```python
from build123d import *

# Parameters (mm, degrees)
F1_DEPTH = 75
F2_W     = 28
F2_H     = 5.4
F2_W_2   = 28.1193151165
F2_H_2   = 5.3996254659
F2_W_3   = 28.3288413435
F2_H_3   = 5.3951430639
F2_W_4   = 28.8207556829
F2_W_5   = 28.5256083831
F2_H_4   = 5.4125102987
F2_W_6   = 29.607820116
F2_W_7   = 29.9029674158
F3_DEPTH = 2.8
F5_DEPTH = 5
F6_R     = 1.6
F7_DEPTH = 3.101
F8_SIZE  = 2
F9_R     = 0.5


with BuildPart() as f1:
    # F0 (on Front) → F1 (new body, symmetric)
    with BuildSketch(Plane.XZ):
        Polygon((-7.5, -4.8), (7.5, -4.8), (7.5, -3), (10.5, 0.3), (7.5, 3.3), (-7.5, 3.3), (-10.5, 0.3), (-7.5, -3), align=None)
    extrude(amount=F1_DEPTH, both=True)

    # F2 (on face) → F3 (cut)
    with BuildSketch(Plane.XY.offset(3.3)):
        Rectangle(F2_W, F2_H)
        with Locations((0.0596575582, 9.8198127329)):
            Rectangle(F2_W_2, F2_H_2)
        with Locations((0.1644206718, 19.6375715319)):
            Rectangle(F2_W_3, F2_H_3)
        with Locations((0.4103778414, 29.46)):
            Rectangle(F2_W_4, F2_H)
        with Locations((0.2628041916, -9.8137448507)):
            Rectangle(F2_W_5, F2_H_4)
        with Locations((0.803910058, -19.6274897013)):
            Rectangle(F2_W_6, F2_H)
        with Locations((0.9514837079, -29.4474897013)):
            Rectangle(F2_W_7, F2_H)
        with Locations((0.4103778414, 39.28)):
            Rectangle(F2_W_4, F2_H)
        with Locations((0.4103778414, 49.1)):
            Rectangle(F2_W_4, F2_H)
        with Locations((0.9514837079, -39.2674897013)):
            Rectangle(F2_W_7, F2_H)
        with Locations((0.9514837079, -49.0874897013)):
            Rectangle(F2_W_7, F2_H)
    extrude(amount=-F3_DEPTH, mode=Mode.SUBTRACT)

    # F4 (on face) → F5 (cut)
    with BuildSketch(Plane.XY.offset(3.3)):
        with BuildLine():
            Line((-4.9999021515, -71), (-4.9999021515, -73))
            Line((-4.9999021515, -73), (-4.9999021515, -75))
            Line((-4.9999021515, -75), (5, -75))
            Line((5, -75), (5, -73))
            Line((5, -73), (5, -71))
            ThreePointArc((5, -71), (4.89242e-05, -66.0000489242), (-4.9999021515, -71))
        make_face()
        with BuildLine():
            ThreePointArc((-4.9999021515, 71), (4.89242e-05, 65.9778812301), (5, 71))
            Line((5, 71), (5, 73))
            Line((5, 73), (5, 75))
            Line((5, 75), (-4.9999021515, 75))
            Line((-4.9999021515, 75), (-4.9999021515, 73))
            Line((-4.9999021515, 73), (-4.9999021515, 71))
        make_face()
    extrude(amount=-F5_DEPTH, mode=Mode.SUBTRACT)

    # F6 (on face) → F7 (cut, through all)
    with BuildSketch(Plane.XY.offset(-1.7)):
        with Locations((0, -70.6000489272)):
            Circle(F6_R)
        with Locations((0, 70.5778812331)):
            Circle(F6_R)
    extrude(amount=-F7_DEPTH, mode=Mode.SUBTRACT)

    # F8
    f8_edges = [f1.edges().sort_by_distance(p)[0] for p in [
        (9, 75, 1.8),
        (-9, 75, 1.8),
        (9, -75, 1.8),
        (-9, -75, 1.8),
    ]]
    chamfer(f8_edges, length=F8_SIZE)

    # F9
    f9_edges = [f1.edges().sort_by_distance(p)[0] for p in [
        (-7.5, 24.547572, 3.3),
        (-7.5, 14.729813, 3.3),
        (-7.5, 4.91, 3.3),
        (-7.5, -4.903745, 3.3),
        (-7.5, -14.723745, 3.3),
        (-7.5, -24.53749, 3.3),
        (7.5, -24.53749, 3.3),
        (7.5, -14.723745, 3.3),
        (7.5, 4.91, 3.3),
        (7.5, 14.729813, 3.3),
        (7.5, 24.547572, 3.3),
        (-7.076516, 75, 0.895057),
        (9, 73, 1.8),
        (-9, 73, 1.8),
        (7.076565, -75, 0.895008),
        (9, -73, 1.8),
        (-7.076516, -75, 0.895057),
        (-9, -73, 1.8),
        (-7.5, -75, -3.9),
        (7.5, -75, -3.9),
        (7.5, 75, -3.9),
        (-7.5, 75, -3.9),
    ]]
    fillet(f9_edges, radius=F9_R)


solid = f1.part
```
Work out the finished part from the listing and answer in its coordinate system (mm). A direction names the side the tool comes from. Round coordinates to 2 decimals unless told otherwise and drop trailing zeros. Order: outer loops, then holes, each group sorted by start corner. A loop starts at its lowest first (then second) coordinate and runs counter-clockwise, first axis right, second up.
Q1. Find the intervals of material crossed by line 1 along Y through (x, z) = (0, -3.5); line 2 along X through (y, z) = (23.5, -3.5); line 3 along Z through (x, y) = (6.5, -29.5), in increasing order.
Solution:
line 1: y = -75 to -72.2, -69 to 68.98, 72.18 to 75
line 2: x = -7.5 to 7.5
line 3: z = -4.8 to 0.5
Q2. Given pin 1 Ø2 at (y, z) = (17, 0.5) entering from -X; pin 2 Ø0.5 at (y, z) = (-29.5, -3.5) entering from +X; pin 3 Ø3 at (x, z) = (-2.5, 0.5) entering from +Y, each flat-ended and moving along its own axis, determine where each tip first touches the part or whether it passes through.
Solution:
pin 1: stops at x = -10.5
pin 2: stops at x = 7.5
pin 3: stops at y = 67.98
Q3. A cutting plane is placed at B-B, the plane x = 0. Count the separate pieces of the cut face and the enclosed holes in it, then the cut area to 3 significant figures.
Solution:
separate pieces: 3
enclosed holes: 0
area: 939 mm2
Q4. A cutting plane is placed at A-A, the plane y = 4.5. Determine the outline of the cut face in (x, z).
Solution:
outline: (-10.5, 0.3) - (-7.5, -3) - (-7.5, -4.8) - (7.5, -4.8) - (7.5, -3) - (10.5, 0.3) - (7.65, 3.15) arc R0.5 ccw to (7.29, 3.3) - (-7.29, 3.3) arc R0.5 ccw to (-7.65, 3.15) - close
Q5. The mould has two halves that part along Y. Classify faces 1 (the flat face through (0, 32.16, 2)), 2 (the cylindrical face through (6.99, -74.96, 0.96)), 3 (the flat face through (0, -34, 3.3)): pulls with the +Y half, pulls with the -Y half, needs draft (parallel to the pull), parting line crosses it, or undercut.
Solution:
face 1: undercut
face 2: pulls with the -Y half
face 3: needs draft
Q6. A tool of negligible diameter and unlimited length cuts with its end or side. For faces 4 (the flat face through (0, -41.967, 2)), 5 (the cylindrical face through (8.903, -72.982, 1.845)), 6 (the cylindrical face through (0, -66, 1)), from which of +Z, -Z, +X, -X, +Y, -Y can it reach the whole face along a straight path? Write none if from no direction.
Solution:
face 4: +Z, +X, -X
face 5: +Z, +X, -Y
face 6: +Z, -Y
Q7. A cutting plane is placed at C-C, the plane y = 60. Determine the outline of the cut face in (x, z).
Solution:
outline: (-10.5, 0.3) - (-7.5, -3) - (-7.5, -4.8) - (7.5, -4.8) - (7.5, -3) - (10.5, 0.3) - (7.5, 3.3) - (-7.5, 3.3) - close
